Model file for the job. Use its own axes, mm. A direction names the side the tool comes from. Round coordinates to 2 decimals unless told otherwise and drop trailing zeros. Loops run counter-clockwise (first coordinate to the right, second up) from the corner with the lowest first, then second, coordinate; pieces in that order, holes last. Notation, with made-up numbers: (79.25, 83) - (115.25, 83) arc R19 cw to (115.25, 103) - close; hole circle Ø2 at (40.25, 55.5). An arc over 180 degrees is marked (long way). Use one line per item in the form item = value.
Autodesk Inventor part; units mm, degrees
ref_plane "YZ Plane" through (0, 0, 0) normal (1, 0, 0) x (0, 1, 0)
ref_plane "XZ Plane" through (0, 0, 0) normal (0, 1, 0) x (-1, 0, 0)
ref_plane "XY Plane" through (0, 0, 0) normal (0, 0, 1) x (1, 0, 0)
sketch "Sketch1" plane through (0, 0, 0) normal (0, 0, 1) x (1, 0, 0)
  line L0 (0, 0) -> (-14, 0) construction
  circle A0 centre (-14, 0) radius 4
  circle A1 centre (0, 0) radius 4
  line L1 (12, -9) -> (-26, -9)
  line L2 (-26, -9) -> (-26, 9)
  line L3 (-26, 9) -> (12, 9)
  line L4 (12, 9) -> (12, -9)
  line L5 (12, -9) -> (-26, 9) construction
  line L6 (-26, -9) -> (12, 9) construction
  point P0 (-7, 0)
  dimension "d0" = 8
  dimension "d1" = 14
  dimension "d2" = 12
  dimension "d3" = 18
  dimension "d13" = 38
extrude "Extrusion1" add sketch "Sketch1" along normal blind 10
sketch "Sketch2" plane through (-26, 9, 0) normal (0, 1, 0) x (1, 0, 0)
  circle A0 centre (19.5, -5) radius 2.5
  line L0 (19.5, -5) -> (0, -5) construction
  line L1 (0, 0) -> (0, -10) construction
  point P0 (26, 0)
  dimension "d6" = 5
  dimension "d17" = 19.5
extrude "Extrusion2" cut sketch "Sketch2" against normal through all
fillet "Fillet1" radius 6 4 edges at (12, 9, 5) (-26, 9, 5) (-26, -9, 5) (12, -9, 5)
sketch "Sketch3" plane through (0, 0, 10) normal (0, 0, 1) x (1, 0, 0)
  line L0 (-20, -9) -> (6, -9)
  circle A0 centre (0, 0) radius 4
  circle A1 centre (-14, 0) radius 4
  line L1 (-14, 0) -> (0, 0) construction
  line L2 (0, -0.75) -> (-14, -0.75)
  line L3 (-14, -0.75) -> (-14, 0.75)
  line L4 (-14, 0.75) -> (0, 0.75)
  line L5 (0, 0.75) -> (0, -0.75)
  line L6 (0, -0.75) -> (-14, 0.75) construction
  line L7 (-14, -0.75) -> (0, 0.75) construction
  point P0 (-7, 0)
  dimension "d10" = 1.5
extrude "Extrusion3" cut sketch "Sketch3" against normal through all contours L4 L5 L2 A0 | A0 L2 A1 L4 | A1 L2 L3 L4 picked at (-1.3307, -0.0838) picked at (-12.6667, 0)
sketch "Sketch4" plane through (0, 0, 10) normal (0, 0, 1) x (1, 0, 0)
  line L0 (-10.0709, 0.75) -> (-3.9291, 0.75) construction
  arc A0 (-3.9291, -0.75) -> (-3.9291, 0.75) centre (0, 0) ccw construction
  line L1 (-3.9291, -0.75) -> (-10.0709, -0.75) construction
  arc A1 (-10.0709, 0.75) -> (-10.0709, -0.75) centre (-14, 0) ccw construction
  arc A2 (6, -9) -> (12, -3) centre (6, -3) ccw construction
  line L2 (12, -3) -> (12, 3) construction
  arc A3 (12, 3) -> (6, 9) centre (6, 3) ccw construction
  line L3 (6, 9) -> (-20, 9) construction
  arc A4 (-20, 9) -> (-26, 3) centre (-20, 3) ccw construction
  line L4 (-26, 3) -> (-26, -3) construction
  arc A5 (-26, -3) -> (-20, -9) centre (-20, -3) ccw construction
  line L5 (-20, -9) -> (6, -9) construction
  line L6 (-9.2375, -4.7625) -> (-18.7625, -4.7625)
  line L7 (-18.7625, -4.7625) -> (-18.7625, 4.7625)
  line L8 (-18.7625, 4.7625) -> (-9.2375, 4.7625)
  line L9 (-9.2375, 4.7625) -> (-9.2375, -4.7625)
  line L10 (-9.2375, -4.7625) -> (-18.7625, 4.7625) construction
  line L11 (-18.7625, -4.7625) -> (-9.2375, 4.7625) construction
  dimension "d14" = 9.525
extrude "Extrusion4" cut sketch "Sketch4" against normal through all
properties part number "crank web"
1. Tool access for faces 1 (the flat face through (-14, 4.762, 5)), 2 (the cylindrical face through (10.289, 7.196, 5.07)): list every direction of +Z, -Z, +X, -X, +Y, -Y with a clear straight run to the whole face (end or side of a thin tool).
Geometry check:
face_1 = +Z, -Z
face_2 = +Z, -Z, +X, +Y
2. Cut at B-B, the plane x = -8. Give the cut face in (y, z), plus the area to 3 significant figures.
Geometry check:
outline = (-9, 0) - (-0.75, 0) - (-0.75, 3) - (-9, 3) - close; (-9, 7) - (-0.75, 7) - (-0.75, 10) - (-9, 10) - close; (0.75, 0) - (9, 0) - (9, 3) - (0.75, 3) - close; (0.75, 7) - (9, 7) - (9, 10) - (0.75, 10) - close
area = 99.0 mm^2
3. Wall check: probe 1 along Y at (x, z) = (-18.5, 5); probe 2 along Z at (x, y) = (-6.5, -7); probe 3 along Y at (x, z) = (0, 2.75). Give the ranges that are in metal, low to high.
Geometry check:
probe_1 = -9 to -4.76, 4.76 to 9
probe_2 = 0 to 2.5, 7.5 to 10
probe_3 = -9 to -4, 4 to 9
4. Cut at D-D, the plane z = 8.5. Give the cut face in (x, y).
Geometry check:
outline = (-26, -3) arc R6 ccw to (-20, -9) - (6, -9) arc R6 ccw to (12, -3) - (12, 3) arc R6 ccw to (6, 9) - (-20, 9) arc R6 ccw to (-26, 3) - close; hole (-18.76, -4.76) - (-9.24, -4.76) - (-9.24, -0.75) - (-3.93, -0.75) arc R4 ccw (long way) to (-3.93, 0.75) - (-9.24, 0.75) - (-9.24, 4.76) - (-18.76, 4.76) - close
5. Flat gauge pin, fed straight in: pin 1 (3 mm diameter, centred on x = -6.5, z = 5, fed in from -Y). Where does the tip first touch, or does it go through?
Geometry check:
pin_1 = through
6. Cut at A-A, the plane z = 5. Give the cut face in (x, y), plus the area to 3 significant figures.
Geometry check:
outline = (-26, -3) arc R6 ccw to (-20, -9) - (-9, -9) - (-9, -0.75) - (-9.24, -0.75) - (-9.24, -4.76) - (-18.76, -4.76) - (-18.76, 4.76) - (-9.24, 4.76) - (-9.24, 0.75) - (-9, 0.75) - (-9, 9) - (-20, 9) arc R6 ccw to (-26, 3) - close; (-4, -9) - (6, -9) arc R6 ccw to (12, -3) - (12, 3) arc R6 ccw to (6, 9) - (-4, 9) - (-4, 0.75) - (-3.93, 0.75) arc R4 cw (long way) to (-3.93, -0.75) - (-4, -0.75) - close
area = 422 mm^2
7. Cut at C-C, the plane y = -3.5. Give the cut face in (x, z).
Geometry check:
outline = (-25.98, 0) - (-18.76, 0) - (-18.76, 10) - (-25.98, 10) - close; (-9.24, 0) - (-1.94, 0) - (-1.94, 10) - (-9.24, 10) - close; (1.94, 0) - (11.98, 0) - (11.98, 10) - (1.94, 10) - close; hole circle Ø5 at (-6.5, 5)
8. Pull direction X, two halves, no side cores. Call faces 3 (the flat face through (-10, 9, 5)), 4 (the flat face through (-26, 0, 5)), 5 (the flat face through (-9.238, 3, 5)): +X half, -X half, draft (parallel to the pull), parting line (faces both ways), or undercut.
Geometry check:
face_3 = draft
face_4 = -X half
face_5 = undercut
